Could you check a few things on this model? Use its own coordinates, in mm. A direction names the side the tool comes from. Round coordinates to 2 decimals unless told otherwise and drop trailing zeros. Loops run counter-clockwise (first coordinate to the right, second up) from the corner with the lowest first, then second, coordinate; pieces in that order, holes last. Notation, with made-up numbers: (-34.75, 9) -> (-5.75, 9) arc R38 ccw to (-5.75, 48) -> close; hole circle Ø9 at (61, 4). An arc over 180 degrees is marked (long way). Put each result on its own line as item: value. Start each with the question number.
1. Imagine slicing it at B-B, the plane y = -48.5. Please give me the cut outline in (x, z), and give its area (3 significant figures).
2. I'm going to push flat-ended pins straight in: P1, Ø1.5, axis at y = 43, z = 44.5, coming from the +X side; P2, Ø1.5, axis at x = 28, z = 9.5, coming from the +Y side; P3, Ø2, axis at x = 45.5, z = 45, coming from the +Y side. Where does each tip first touch, or does it pass through?
3. I need wall thicknesses on line 1 (Y direction, x = -71, z = 5.5); line 2 (Y direction, x = 45, z = 22); line 3 (Y direction, x = 83, z = 6.5). Which ranges of each line are inside material? Lowest first, please. Write a range as [from, to].
4. Which directions (+Z, -Z, +X, -X, +Y, -Y) give clear straight access to the entire face, cutting with the end or side of a thin tool? Please do faces 5 (the flat face through (-98, 5, 27)), 6 (the flat face through (-70, 70, 27)), 7 (the flat face through (-5, -98, 27)), 8 (the flat face through (-65.985, 73.056, 26.65)), 9 (the flat face through (99, 0, 27)).
5. If we mould it in two halves opening along Y, with no side actions, what happens to faces 1 (the flat face through (65.985, -73.056, 26.65)), 2 (the cylindrical face through (-33.4, 88.4, 26.6)), 3 (the flat face through (70, -70, 27)), 4 (the flat face through (16, 92, 52))? For each: pulls with the +Y half, pulls with the -Y half, needs draft (parallel to the pull), parting line crosses it, or undercut.
```python
from build123d import *
from build123d.topology import SkipClean

# Parameters (mm, degrees)
SKETCH1_R           = 102.5
SKETCH1_R_2         = 92.5
BOSS_EXTRUDE1_DEPTH = 2
SKETCH2_R           = 94.5
SKETCH2_R_2         = 92.5
BOSS_EXTRUDE2_DEPTH = 50
BOSS_EXTRUDE3_DEPTH = 50
CIRPATTERN1_COUNT   = 8


with BuildPart() as part:
    # Sketch1 → Boss-Extrude1 (new body)
    with BuildSketch(Plane.XY):
        Circle(SKETCH1_R)
        Circle(SKETCH1_R_2, mode=Mode.SUBTRACT)
    extrude(amount=BOSS_EXTRUDE1_DEPTH)

    # Sketch2 → Boss-Extrude2 (add)
    with BuildSketch(Plane.XY.offset(2)):
        Circle(SKETCH2_R)
        Circle(SKETCH2_R_2, mode=Mode.SUBTRACT)
    extrude(amount=BOSS_EXTRUDE2_DEPTH)

    # Sketch3 → Boss-Extrude3 (add)
    with BuildSketch(Plane.XY.offset(2)):
        with BuildLine():
            Line((0, 102.5), (0, 94.5))
            ThreePointArc((0, 94.5), (2.500875909, 94.466902245), (5, 94.367632163))
            Line((5, 94.367632163), (5, 102.377976147))
            ThreePointArc((5, 102.377976147), (2.50074438, 102.469489496), (0, 102.5))
        make_face()
    boss_extrude3 = extrude(amount=BOSS_EXTRUDE3_DEPTH)

    # CirPattern1: Boss-Extrude3 ×8 about axis
    with SkipClean():  # the faces are left unmerged after this step: merging them gives an invalid solid
        cirpattern1_axis = Axis((0, 0, 0), (0, 0, 1))
        for i in range(1, CIRPATTERN1_COUNT):
            add(boss_extrude3.rotate(cirpattern1_axis, i * 360 / CIRPATTERN1_COUNT))


solid = part.part
```
Entries:
1. outline: (-90.3, 0) -> (-78.77, 0) -> (-78.77, 52) -> (-81.1, 52) -> (-81.1, 2) -> (-90.3, 2) -> close; (78.77, 0) -> (90.3, 0) -> (90.3, 2) -> (81.1, 2) -> (81.1, 52) -> (78.77, 52) -> close
1. area: 280 mm^2
2. P1: x = 84.53
2. P2: y = 90.49
2. P3: y = 83.37
3. line 1: [-71, -63.93], [-62.36, -59.29], [59.29, 62.36], [71, 73.93]
3. line 2: [-83.1, -80.82], [80.82, 83.1]
3. line 3: [-45.18, -40.83], [40.83, 45.18]
4. face 5: +Z, -X, +Y
4. face 6: +Z, -X
4. face 7: +Z, -X, -Y
4. face 8: +Z, +Y
4. face 9: +Z, +X, +Y
5. face 1: pulls with the -Y half
5. face 2: pulls with the +Y half
5. face 3: undercut
5. face 4: needs draft
